Geometry check sheet. Reference: the model listing, model coordinates, mm. A direction names the side the tool comes from. Give positions to 0.01 mm unless a question says otherwise; leave off trailing zeros. Order: outer loops, then holes, each group sorted by start corner. A loop starts at its lowest first (then second) coordinate and runs counter-clockwise, first axis right, second up.
from build123d import *

# Parameters (mm, degrees)
SKETCH1_W           = 16.28
SKETCH1_H           = 6
BOSS_EXTRUDE1_DEPTH = 4
CUT_EXTRUDE1_DEPTH  = 3
SKETCH4_W           = 0.5
SKETCH4_H           = 0.5
BOSS_EXTRUDE2_DEPTH = 3


with BuildPart() as part:
    # Sketch1 → Boss-Extrude1 (new body)
    with BuildSketch(Plane(origin=(0, 0, 0), x_dir=(1, 0, 0), z_dir=(0, 1, 0))):
        Rectangle(SKETCH1_W, SKETCH1_H)
    extrude(amount=BOSS_EXTRUDE1_DEPTH)

    # Sketch2 → Cut-Extrude1 (cut)
    with BuildSketch(Plane(origin=(0, 4, 0), x_dir=(1, 0, 0), z_dir=(0, 1, 0))):
        Polygon((-7.64, -2.5), (-7.64, 1), (7.64, 1), (7.64, -2.5), (4, -2.5), (4, -3), (-4, -3), (-4, -2.5), align=None)
    extrude(amount=-CUT_EXTRUDE1_DEPTH, mode=Mode.SUBTRACT)

    # Sketch4 → Boss-Extrude2 (add)
    with BuildSketch(Plane(origin=(0, 1, 0), x_dir=(1, 0, 0), z_dir=(0, 1, 0))):
        with Locations((-3, -0.881352283)):
            Rectangle(SKETCH4_W, SKETCH4_H)
        with Locations((-5, -0.881352283)):
            Rectangle(SKETCH4_W, SKETCH4_H)
        with Locations((-1, -0.881352283)):
            Rectangle(SKETCH4_W, SKETCH4_H)
        with Locations((1, -0.881352283)):
            Rectangle(SKETCH4_W, SKETCH4_H)
        with Locations((3, -0.881352283)):
            Rectangle(SKETCH4_W, SKETCH4_H)
        with Locations((5, -0.881352283)):
            Rectangle(SKETCH4_W, SKETCH4_H)
    extrude(amount=BOSS_EXTRUDE2_DEPTH)


solid = part.part
Item 1: Gauge pin test, flat ends, axial feed: pin 1 (1 mm diameter, centred on x = -2, z = 0, fed in from -Y); pin 2 (1 mm diameter, centred on x = -2.5, y = 2, fed in from +Z). Record the tip position at first contact, or that the pin passes through.
Reported:
pin 1: stops at y = 0
pin 2: stops at z = 1.13
Item 2: Sectioned sample at D-D (x = -2.25). Enter the section's corners in (y, z).
Reported:
outline: (0, -3) - (4, -3) - (4, -1) - (1, -1) - (1, 3) - (0, 3) - close
Item 3: Sectioned sample at B-B (x = -5). Enter the section's corners in (y, z), and give its area (3 significant figures).
Reported:
outline: (0, -3) - (4, -3) - (4, -1) - (1, -1) - (1, 0.63) - (4, 0.63) - (4, 1.13) - (1, 1.13) - (1, 2.5) - (4, 2.5) - (4, 3) - (0, 3) - close
area: 15.0 mm2
Item 4: Scan lines: L1, parallel to X at y = 1.85, z = 1.6; L2, parallel to Z at x = 4.25, y = 3.05; L3, parallel to Y at x = 6.75, z = 1.45. Record each from-to range of solid material in increasing order.
Reported:
L1: x = -8.14 to -7.64, 7.64 to 8.14
L2: z = -3 to -1, 2.5 to 3
L3: y = 0 to 1
Item 5: Draft check along Z on faces 1 (the flat face through (-7.64, 3, 1)), 2 (the flat face through (-0.1, 4, -1.4)), 3 (the flat face through (0, 2, -3)). Enter one of: released by +Z, released by -Z, zero draft, split by the parting line, or undercut.
Reported:
face 1: undercut
face 2: zero draft
face 3: released by -Z
Item 6: Sectioned sample at C-C (y = 2.05). Give the number of separate pieces and of enclosed holes in the cut face, and give its area (3 significant figures).
Reported:
separate pieces: 7
enclosed holes: 0
area: 41.7 mm2
Item 7: Sectioned sample at A-A (z = -0.05). Enter the section's corners in (x, y).
Reported:
outline: (-8.14, 0) - (8.14, 0) - (8.14, 4) - (7.64, 4) - (7.64, 1) - (-7.64, 1) - (-7.64, 4) - (-8.14, 4) - close
Item 8: Set-up check for faces 4 (the flat face through (6, 3, 2.5)), 5 (the flat face through (-8.14, 2, 0)): record each of +Z, -Z, +X, -X, +Y, -Y from which the full face is reachable in a straight line by a thin tool's end or side.
Reported:
face 4: +Y
face 5: +Z, -Z, -X, +Y, -Y
